Source: three-view drawing plus pictorial views. Frame: mm from the lowest corner of the part. Round coordinates to 2 decimals unless told otherwise and drop trailing zeros. Write each loop counter-clockwise with the first axis right and the second up, starting at its lowest first coordinate (ties: lowest second). Pieces come first, ordered by that corner, then holes.
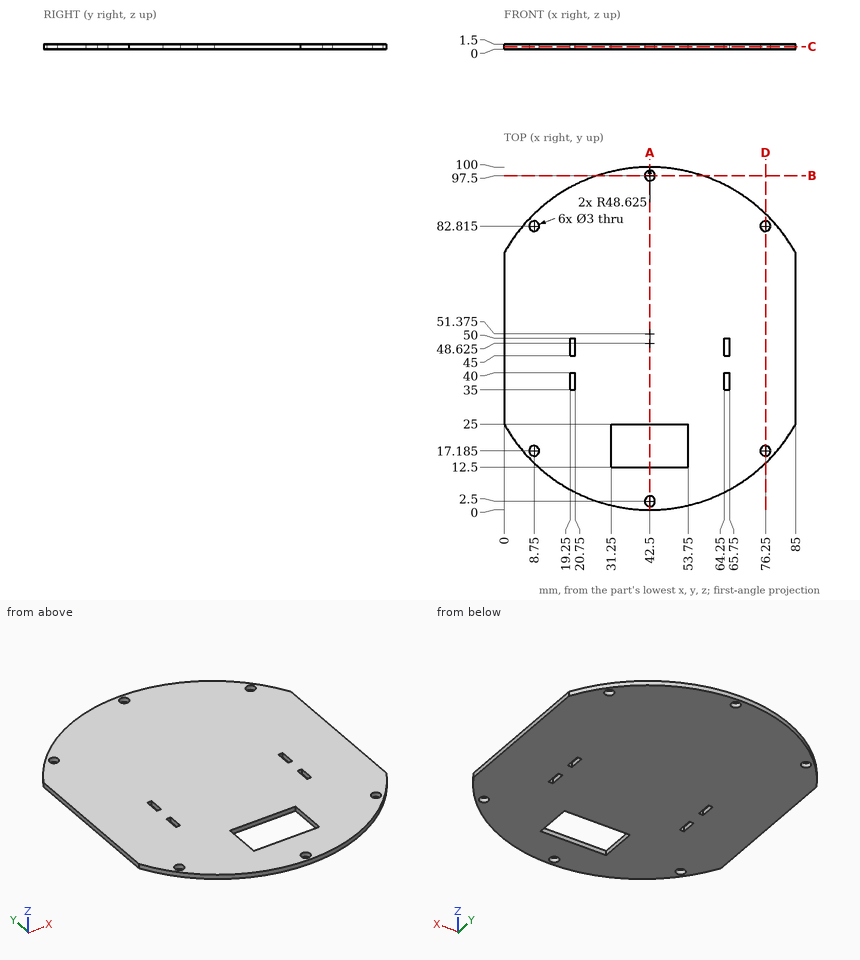
1) Section D-D on x = 76.25. Output: boundary loops of the cut face in (y, z) (1 decimal), plus the area to 3 significant figures.
2) First-contact query: P1, Ø0.8, axis at x = 42.5, z = 1, coming from the +Y side; P2, Ø0.8, axis at x = 41, z = 0.5, coming from the -Y side. Flat tips, straight axial feed; report the tip coordinate or a pass-through.
3) Section C-C on z = 0.7. State how many separate pieces and enclosed holes the cut face has, plus the area to 3 significant figures.
4) Line query: probe 1 along X at (y, z) = (47.5, 0.95); probe 2 along Y at (x, z) = (42.5, 0.9); probe 3 along Y at (x, z) = (8.75, 1) (1 decimal). Output: solid intervals per line, ascending.
5) Section B-B on y = 97.5. Output: boundary loops of the cut face in (x, z).
6) Section A-A on x = 42.5. Output: boundary loops of the cut face in (y, z).
Filled in:
1. outline: (13.6, 0) - (15.7, 0) - (15.7, 1.5) - (13.6, 1.5) - close; (18.7, 0) - (81.3, 0) - (81.3, 1.5) - (18.7, 1.5) - close; (84.3, 0) - (86.4, 0) - (86.4, 1.5) - (84.3, 1.5) - close
1. area: 100 mm2
2. P1: stops at y = 100
2. P2: stops at y = 0.01
3. separate pieces: 1
3. enclosed holes: 11
3. area: 6,920 mm2
4. probe 1: x = 0 to 19.25, 20.75 to 64.25, 65.75 to 85
4. probe 2: y = 0 to 1, 4 to 12.5, 25 to 96, 99 to 100
4. probe 3: y = 13.6 to 15.7, 18.7 to 81.3, 84.3 to 86.4
5. outline: (27.11, 0) - (41, 0) - (41, 1.5) - (27.11, 1.5) - close; (44, 0) - (57.89, 0) - (57.89, 1.5) - (44, 1.5) - close
6. outline: (0, 0) - (1, 0) - (1, 1.5) - (0, 1.5) - close; (4, 0) - (12.5, 0) - (12.5, 1.5) - (4, 1.5) - close; (25, 0) - (96, 0) - (96, 1.5) - (25, 1.5) - close; (99, 0) - (100, 0) - (100, 1.5) - (99, 1.5) - close
